Could you check a few things on this model? Use its own coordinates, in mm. Face numbers are marked on the shaded views. A direction names the side the tool comes from. Give positions to 0.01 mm unless a question says otherwise; leave off trailing zeros. Order: outer loops, then holes, each group sorted by start corner. A loop starts at its lowest first (then second) coordinate and runs counter-clockwise, first axis right, second up.
(1) Imagine slicing it at B-B, the plane y = -5. Write out the boundary of the cut face in (x, z), then the cut area to 3 significant figures.
(2) Imagine slicing it at D-D, the plane x = -8. Write out the boundary of the cut face in (y, z) (3 decimals).
(3) On a 3-axis mill with a long thin cutter (end or side, diameter ignored), from which of +Z, -Z, +X, -X, +Y, -Y can I reach the whole of each face in a straight line? I mean the marked faces 4, 5, 6 and 7. Say none if no direction works.
(4) If I drill on probe 1 along Y at (x, z) = (13.52, 9.25); probe 2 along Y at (x, z) = (13.5, 11.25); probe 3 along Y at (x, z) = (-19, 7.25) (3 decimals), over which ranges is the centre line in solid material (lowest first)?
(5) Imagine slicing it at C-C, the plane z = 8.25. Write out the boundary of the cut face in (x, y) (3 decimals), then the cut area to 3 significant figures.
(6) Imagine slicing it at A-A, the plane x = 13.52. Write out the boundary of the cut face in (y, z) (3 decimals).
(7) If we mould it in two halves opening along Y, with no side actions, what happens to the marked faces 1, 2 and 3? For each: released by +Y, released by -Y, zero draft, split by the parting line, or undercut.
(8) Will these pins go through, and if not, where does the flat tip stop? pin 1 (1.5 mm diameter, centred on x = 0.5, y = -12, fed in from +Z) (3 decimals); pin 2 (5.5 mm diameter, centred on x = 3.5, y = 12.5, fed in from +Z).
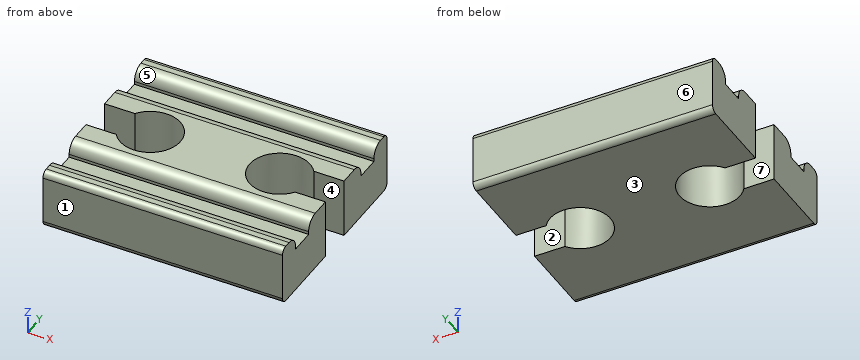
from build123d import *

# Parameters (mm, degrees)
F0_W     = 50
F0_H     = 40.6
F1_DEPTH = 12.5
F3_DEPTH = 12.501
F4_W     = 50
F4_H     = 5.08
F5_DEPTH = 3.175
F6_R     = 1.27
F7_R     = 2.54


# Not quite as in the source:
# - a pattern or mirror of a feature is missing from the dataset's text; its kind, count and spacing are read off the source's solid


with BuildPart() as f1:
    # F0 (on Top) → F1 (new body)
    with BuildSketch(Plane.XY):
        Rectangle(F0_W, F0_H)
    extrude(amount=F1_DEPTH)

    # F2 (on Top) → F3 (cut, through all)
    with BuildSketch(Plane.XY):
        with BuildLine():
            Line((25, -2.794), (25, 3.625))
            Line((25, 3.625), (18.6726085627, 3.625))
            ThreePointArc((18.6726085627, 3.625), (7.22, 0), (18.6726085627, -3.625))
            Line((18.6726085627, -3.625), (25, -3.625))
            Line((25, -3.625), (25, -2.794))
        make_face()
    f3 = extrude(amount=F3_DEPTH, mode=Mode.SUBTRACT)

    # F3_copies: F3 across plane
    add(f3.mirror(Plane(origin=(0, 0, 0), x_dir=(0, 0, -1), z_dir=(-1, 0, 0))), mode=Mode.SUBTRACT)

    # F4 (on face) → F5 (cut)
    with BuildSketch(Plane.XY.offset(12.5)):
        with Locations((0, 12.68)):
            Rectangle(F4_W, F4_H)
    f5 = extrude(amount=-F5_DEPTH, mode=Mode.SUBTRACT)

    # F5_copies: F5 across plane
    add(f5.mirror(Plane(origin=(0, 0, 0), x_dir=(0, 0, -1), z_dir=(0, -1, 0))), mode=Mode.SUBTRACT)

    # F6
    f6_edges = [f1.edges().sort_by_distance(p)[0] for p in [
        (0, 20.3, 12.5),
        (0, -20.3, 12.5),
        (0, 20.3, 0),
        (0, -20.3, 0),
    ]]
    fillet(f6_edges, radius=F6_R)

    # F7
    f7_edges = [f1.edges().sort_by_distance(p)[0] for p in [
        (0, 15.22, 12.5),
        (0, 10.14, 12.5),
        (0, -10.14, 12.5),
        (0, -15.22, 12.5),
    ]]
    fillet(f7_edges, radius=F7_R)


solid = f1.part
Answer block:
1. outline: (-25, 0) - (-17.35, 0) - (-17.35, 12.5) - (-25, 12.5) - close; (-9.69, 0) - (9.69, 0) - (9.69, 12.5) - (-9.69, 12.5) - close; (17.35, 0) - (25, 0) - (25, 12.5) - (17.35, 12.5) - close
1. area: 433 mm2
2. outline: (-20.3, 1.27) arc R1.27 ccw to (-19.03, 0) - (-3.036, 0) - (-3.036, 12.5) - (-7.6, 12.5) arc R2.54 ccw to (-10.14, 9.96) - (-10.14, 9.325) - (-15.22, 9.325) - (-15.22, 9.96) arc R2.54 ccw to (-17.76, 12.5) - (-19.03, 12.5) arc R1.27 ccw to (-20.3, 11.23) - close; (3.036, 0) - (19.03, 0) arc R1.27 ccw to (20.3, 1.27) - (20.3, 11.23) arc R1.27 ccw to (19.03, 12.5) - (17.76, 12.5) arc R2.54 ccw to (15.22, 9.96) - (15.22, 9.325) - (10.14, 9.325) - (10.14, 9.96) arc R2.54 ccw to (7.6, 12.5) - (3.036, 12.5) - close
3. face 4: +Z, -Z, +X
3. face 5: +Z, +X, -X
3. face 6: +Z, -Z, +X, -X, +Y
3. face 7: +Z, -Z, -X
4. probe 1: y = -20.3 to -6.3, 6.3 to 20.3
4. probe 2: y = -20.3 to -15.57, -9.79 to -6.3, 6.3 to 9.79, 15.57 to 20.3
4. probe 3: y = -20.3 to -3.625, 3.625 to 20.3
5. outline: (-25, -20.3) - (25, -20.3) - (25, -3.625) - (18.673, -3.625) arc R6.3 cw (long way) to (18.673, 3.625) - (25, 3.625) - (25, 20.3) - (-25, 20.3) - (-25, 3.625) - (-18.673, 3.625) arc R6.3 cw (long way) to (-18.673, -3.625) - (-25, -3.625) - close
5. area: 1,700 mm2
6. outline: (-20.3, 1.27) arc R1.27 ccw to (-19.03, 0) - (-6.3, 0) - (-6.3, 12.5) - (-7.6, 12.5) arc R2.54 ccw to (-10.14, 9.96) - (-10.14, 9.325) - (-15.22, 9.325) - (-15.22, 9.96) arc R2.54 ccw to (-17.76, 12.5) - (-19.03, 12.5) arc R1.27 ccw to (-20.3, 11.23) - close; (6.3, 0) - (19.03, 0) arc R1.27 ccw to (20.3, 1.27) - (20.3, 11.23) arc R1.27 ccw to (19.03, 12.5) - (17.76, 12.5) arc R2.54 ccw to (15.22, 9.96) - (15.22, 9.325) - (10.14, 9.325) - (10.14, 9.96) arc R2.54 ccw to (7.6, 12.5) - (6.3, 12.5) - close
7. face 1: released by -Y
7. face 2: undercut
7. face 3: zero draft
8. pin 1: stops at z = 9.325
8. pin 2: stops at z = 11.31
